Verification items for this drawing (mm, ordinates from the low corner). A direction names the side the tool comes from. Give positions to 0.01 mm unless a question says otherwise; leave off trailing zeros. Loops run counter-clockwise (first coordinate to the right, second up) from the corner with the lowest first, then second, coordinate; pieces in that order, holes last. Notation, with made-up numbers: (44, 71.25) -> (101, 71.25) arc R19 ccw to (101, 94.25) -> close; hole circle Ø3 at (-4.5, 61.25). An arc over 180 degrees is marked (long way). Answer as a JSON object with one key per item and string values.
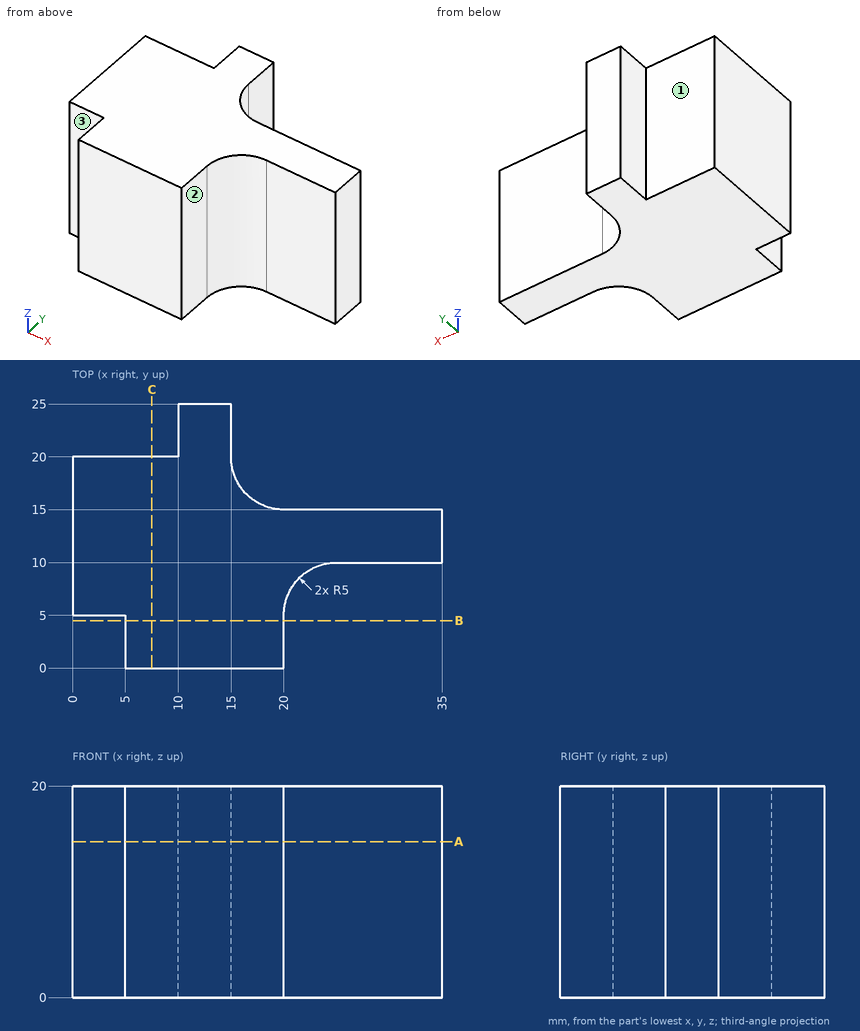
1) Tool access check on the marked faces 1, 2 and 3. Record the directions out of +Z, -Z, +X, -X, +Y, -Y that give a thin tool (end or side, any length) a straight path to the whole face; none if there is none.
Geometry check:
{"face 1": "+Z, -Z, -X, +Y", "face 2": "+Z, -Z, +X, -Y", "face 3": "+Z, -Z, -X, -Y"}
2) Depth check by flat-ended pin: P1, Ø8, axis at x = 32.5, z = 12, coming from the -Y side; P2, Ø1.5, axis at x = 1.5, z = 9, coming from the -Y side; P3, Ø2.5, axis at y = 1.5, z = 12, coming from the -X side. Enter the tip coordinate at first touch or a pass-through.
Geometry check:
{"P1": "stops at y = 10", "P2": "stops at y = 5", "P3": "stops at x = 5"}
3) Material ranges on line 1 along X through (y, z) = (21, 13.75); line 2 along X through (y, z) = (3, 12.75); line 3 along Y through (x, z) = (7.5, 1.75), recorded low to high. Write a range as from..to.
Geometry check:
{"line 1": "x = 10..15", "line 2": "x = 5..20", "line 3": "y = 0..20"}
4) Section check C-C on x = 7.5. Record the cut outline in (y, z).
Geometry check:
{"outline": "(0, 0) -> (20, 0) -> (20, 20) -> (0, 20) -> close"}
5) Section check A-A on z = 14.75. Record the cut outline in (x, y).
Geometry check:
{"outline": "(0, 5) -> (5, 5) -> (5, 0) -> (20, 0) -> (20, 5) arc R5 cw to (25, 10) -> (35, 10) -> (35, 15) -> (20, 15) arc R5 cw to (15, 20) -> (15, 25) -> (10, 25) -> (10, 20) -> (0, 20) -> close"}
6) Section check B-B on y = 4.5. Record the cut outline in (x, z).
Geometry check:
{"outline": "(5, 0) -> (20, 0) -> (20, 20) -> (5, 20) -> close"}
